from build123d import *

# Parameters (mm, degrees)
BOSS_EXTRU_1_DEPTH = 5
ESQUISSE2_R        = 10
BOSS_EXTRU_2_DEPTH = 92
CONG_1_R           = 2


with BuildPart() as part:
    # Esquisse1 → Boss.-Extru.1 (new body)
    with BuildSketch(Plane(origin=(0, 0, 0), x_dir=(1, 0, 0), z_dir=(0, 1, 0))):
        Polygon((-14.767960782, 9.062157753), (-15.232039218, -8.258350323), (-0.464078436, -17.320508076), (14.767960782, -9.062157753), (15.232039218, 8.258350323), (0.464078436, 17.320508076), align=None)
    extrude(amount=BOSS_EXTRU_1_DEPTH)

    # Esquisse2 → Boss.-Extru.2 (add)
    with BuildSketch(Plane(origin=(0, 5, 0), x_dir=(1, 0, 0), z_dir=(0, 1, 0))):
        Circle(ESQUISSE2_R)
    extrude(amount=BOSS_EXTRU_2_DEPTH)

    # Congé1
    cong_1_edges = [part.edges().sort_by_distance(p)[0] for p in [
        (-10, 97, 0),
    ]]
    fillet(cong_1_edges, radius=CONG_1_R)


solid = part.part
Source: CAD feature listing. Evaluate the final solid. Frame: model axes, mm. A direction names the side the tool comes from. Coordinates: 2 decimals unless noted, no trailing zeros. Loops run counter-clockwise (first coordinate to the right, second up) from the corner with the lowest first, then second, coordinate; pieces in that order, holes last. Notation, with made-up numbers: (4, -31.5) - (62, -31.5) arc R23 cw to (62, -15.5) - close; hole circle Ø9 at (6.25, 22). An arc over 180 degrees is marked (long way). Return JSON: item names as keys, results as strings.
Q1. Access query for faces 1 (the flat face through (-7, 5, 7.5)), 2 (the flat face through (0, 0, 0)). Directions: +Z, -Z, +X, -X, +Y, -Y. A direction counts if a zero-diameter tool reaches every point of the face in a straight line with its end or side. Return the directions, or none.
Results:
{"face 1": "+Y", "face 2": "+Z, -Z, +X, -X, -Y"}
Q2. Material intervals for line 1 along Z through (x, y) = (0.5, 37); line 2 along Y through (x, z) = (4, -10); line 3 along X through (y, z) = (34, -2), sorted ascending.
Results:
{"line 1": "-9.99 to 9.99", "line 2": "0 to 5", "line 3": "-9.8 to 9.8"}
Q3. Contact query for flat-ended pins moving along their axis: P1, Ø1, axis at x = -8, z = 10.5, coming from the +Y side; P2, Ø6, axis at x = -2.5, y = 69.5, coming from the +Z side; P3, Ø5, axis at x = -5, y = 54, coming from the -Z side. Output: stop coordinate, or through.
Results:
{"P1": "y = 5", "P2": "z = 10", "P3": "z = -9.68"}
Q4. Section D-D, the plane z = -13. Return loops of the section in (x, y), plus the area to 3 significant figures.
Results:
{"outline": "(-7.5, 0) - (7.5, 0) - (7.5, 5) - (-7.5, 5) - close", "area": "75.0 mm2"}
Q5. Section A-A, the plane y = 20. Return loops of the section in (x, z), plus the area to 3 significant figures.
Results:
{"outline": "circle Ø20 at (0, 0)", "area": "314 mm2"}
Q6. Section B-B, the plane z = 0. Return loops of the section in (x, y), plus the area to 3 significant figures.
Results:
{"outline": "(-15.01, 0) - (15.01, 0) - (15.01, 5) - (10, 5) - (10, 95) arc R2 ccw to (8, 97) - (-8, 97) arc R2 ccw to (-10, 95) - (-10, 5) - (-15.01, 5) - close", "area": "1,990 mm2"}
Q7. Section C-C, the plane x = 12. Return loops of the section in (y, z), plus the area to 3 significant figures.
Results:
{"outline": "(0, -10.24) - (5, -10.24) - (5, 10.56) - (0, 10.56) - close", "area": "104 mm2"}
